Autodesk Inventor part; units mm, degrees
ref_plane "YZ Plane" through (0, 0, 0) normal (1, 0, 0) x (0, 1, 0)
ref_plane "XZ Plane" through (0, 0, 0) normal (0, 1, 0) x (-1, 0, 0)
ref_plane "XY Plane" through (0, 0, 0) normal (0, 0, 1) x (1, 0, 0)
sketch "Sketch1" plane through (0, 0, 0) normal (0, 1, 0) x (-1, 0, 0)
  line L0 (0, 0) -> (50.8, 0)
  line L1 (50.8, 0) -> (50.8, -25.4)
  line L2 (50.8, -25.4) -> (0, -25.4)
  line L3 (0, -25.4) -> (0, 0)
  line L4 (47.625, -22.225) -> (47.625, -3.175)
  line L5 (47.625, -3.175) -> (3.175, -3.175)
  line L6 (3.175, -3.175) -> (3.175, -22.225)
  line L7 (3.175, -22.225) -> (47.625, -22.225)
  dimension "d0" = 25.4
  dimension "d1" = 50.8
  dimension "d2" = 3.175
extrude "Extrusion1" add sketch "Sketch1" along normal blind 571.5
sketch "Sketch2" plane through (-50.8, 0, 0) normal (0, 0, 1) x (1, 0, 0)
  line L0 (0, 0) -> (0, 571.5)
  line L1 (50.8, 0) -> (0, 0)
  line L2 (0, 571.5) -> (50.8, 571.5)
  point P0 (25.4, 25.4)
  point P1 (25.4, 546.1)
  dimension "d5" = 25.4
  dimension "d6" = 25.4
  dimension "d7" = 25.4
  dimension "d8" = 25.4
properties part number "LiftBase-1111-2020"
Could you check a few things on this model? Use its own coordinates, in mm. A direction names the side the tool comes from. Give positions to 0.01 mm unless a question says otherwise; leave off trailing zeros. Order: outer loops, then holes, each group sorted by start corner. A loop starts at its lowest first (then second) coordinate and runs counter-clockwise, first axis right, second up. Notation, with made-up numbers: (43.25, 26) -> (49.25, 26) arc R13 ccw to (49.25, 40) -> close; hole circle Ø2 at (8, 9). An arc over 180 degrees is marked (long way). Answer in a Markdown table with one row per item. Add a question column.
Item 1: For faces 5 (the flat face through (-25, 0, -2)), 6 (the flat face through (-3.175, 282, -13)), which set-ups out of +Z, -Z, +X, -X, +Y, -Y let a thin tool reach every point of the face, with its end or its side?
Item 2: Please list where these lines run through material, in increasing order: probe 1 along Z at (x, y) = (-10.5, 398) (3 decimals); probe 2 along X at (y, z) = (130.5, -4.5) (3 decimals).
Item 3: Imagine slicing it at A-A (x = -10). List the corners of the cut face in (y, z) for me (3 decimals).
Item 4: Imagine slicing it at B-B (z = -8.5). List the corners of the cut face in (x, y) for me (3 decimals), and give its area (3 significant figures).
Item 5: We'd pull the mould along Z, two halves only. Please class faces 1 (the flat face through (-26, 282, -25.4)), 2 (the flat face through (-25, 282, 0)), 3 (the flat face through (-25, 282, -22.225)), 4 (the flat face through (-47.625, 282, -13)): pulls with the +Z half, pulls with the -Z half, needs draft (parallel to the pull), parting line crosses it, or undercut.
Item 6: Imagine slicing it at C-C (y = 411.5). List the corners of the cut face in (x, z) for me (3 decimals), and give its area (3 significant figures).
Result:
| question | item | result |
|---|---|---|
| 1 | face 5 | +Z, -Z, +X, -X, -Y |
| 1 | face 6 | +Y, -Y |
| 2 | probe 1 | -25.4 to -22.225, -3.175 to 0 |
| 2 | probe 2 | -50.8 to -47.625, -3.175 to 0 |
| 3 | outline | (0, -25.4) -> (571.5, -25.4) -> (571.5, -22.225) -> (0, -22.225) -> close; (0, -3.175) -> (571.5, -3.175) -> (571.5, 0) -> (0, 0) -> close |
| 4 | outline | (-50.8, 0) -> (-47.625, 0) -> (-47.625, 571.5) -> (-50.8, 571.5) -> close; (-3.175, 0) -> (0, 0) -> (0, 571.5) -> (-3.175, 571.5) -> close |
| 4 | area | 3,630 mm2 |
| 5 | face 1 | pulls with the -Z half |
| 5 | face 2 | pulls with the +Z half |
| 5 | face 3 | undercut |
| 5 | face 4 | undercut |
| 6 | outline | (-50.8, -25.4) -> (0, -25.4) -> (0, 0) -> (-50.8, 0) -> close; hole (-47.625, -22.225) -> (-3.175, -22.225) -> (-3.175, -3.175) -> (-47.625, -3.175) -> close |
| 6 | area | 444 mm2 |
